Build history of the part. All positions in model axes, mm. Give positions to 0.01 mm unless a question says otherwise; leave off trailing zeros. Order: outer loops, then holes, each group sorted by start corner. A loop starts at its lowest first (then second) coordinate and runs counter-clockwise, first axis right, second up. Notation, with made-up numbers: (48.5, 20) - (63.5, 20) arc R14 cw to (63.5, 28) - close; hole circle Ø9 at (55, 76.25). An arc over 180 degrees is marked (long way). Answer in a Markdown table with one row per item.
```python
from build123d import *

# Parameters (mm, degrees)
SKETCH_1_W             = 5
SKETCH_1_H             = 3.6
EXTRUDE_1_DEPTH        = 50
CUT_EXTRUDE_1_DEPTH    = 101.047438748
SKETCH_3_R             = 1.79995
CUT_EXTRUDE_2_DEPTH    = 0.8
SKETCH_4_R             = 1.2
CUT_EXTRUDE_3_DEPTH    = 51.140702029
FILLET_1_R             = 0.3
FILLET_2_R             = 0.2
CHAMFER_1_SIZE         = 0.25
PATTERN_LINEAR_1_COUNT = 7
PATTERN_LINEAR_1_PITCH = 15


with BuildPart() as part:
    # 草图1 → 凸台-拉伸1 (new, symmetric)
    with BuildSketch(Plane(origin=(0, 0, 0), x_dir=(0, 0, -1), z_dir=(1, 0, 0))):
        Rectangle(SKETCH_1_W, SKETCH_1_H)
    extrude(amount=EXTRUDE_1_DEPTH, both=True)

    # 草图2 → 切除-拉伸1 (cut, through all)
    with BuildSketch(Plane(origin=(50, 0, 0), x_dir=(0, 0, -1), z_dir=(1, 0, 0))):
        with BuildLine():
            Line((2.5, 1.4), (2.5, 0.184))
            ThreePointArc((2.5, 0.184), (2.260324923, 0.318670305), (2.1, 0.542))
            Line((2.1, 0.542), (2, 0.542))
            ThreePointArc((2, 0.542), (1.75, 0.792), (2, 1.042))
            Line((2, 1.042), (2.1, 1.042))
            ThreePointArc((2.1, 1.042), (2.260324923, 1.265329695), (2.5, 1.4))
        make_face()
        with BuildLine():
            Line((-2.1, 1.042), (-2, 1.042))
            ThreePointArc((-2, 1.042), (-1.75, 0.792), (-2, 0.542))
            Line((-2, 0.542), (-2.1, 0.542))
            ThreePointArc((-2.1, 0.542), (-2.260324923, 0.318670305), (-2.5, 0.184))
            Line((-2.5, 0.184), (-2.5, 1.4))
            ThreePointArc((-2.5, 1.4), (-2.260324923, 1.265329695), (-2.1, 1.042))
        make_face()
    extrude(amount=-CUT_EXTRUDE_1_DEPTH, mode=Mode.SUBTRACT)

    # 草图3 → 切除-拉伸2 (cut)
    with BuildSketch(Plane(origin=(0, 1.8, 0), x_dir=(1, 0, 0), z_dir=(0, 1, 0))):
        with Locations(Location((-45, 0, 0), (0, 0, 270))):
            Circle(SKETCH_3_R)
    cut_extrude_2 = extrude(amount=-CUT_EXTRUDE_2_DEPTH, mode=Mode.SUBTRACT)

    # 草图4 → 切除-拉伸3 (cut, through all)
    with BuildSketch(Plane(origin=(0, 1, 0), x_dir=(1, 0, 0), z_dir=(0, 1, 0))):
        with Locations(Location((-45, 0, 0), (0, 0, 270))):
            Circle(SKETCH_4_R)
    cut_extrude_3 = extrude(amount=-CUT_EXTRUDE_3_DEPTH, mode=Mode.SUBTRACT)

    # 圆角1
    fillet_1_edges = [part.edges().sort_by_distance(p)[0] for p in [
        (0, 1.8, 2.5),
        (0, 1.8, -2.5),
    ]]
    fillet(fillet_1_edges, radius=FILLET_1_R)

    # 圆角2
    fillet_2_edges = [part.edges().sort_by_distance(p)[0] for p in [
        (0, 1.4, -2.5),
        (0, 1.042, -2.1),
        (0, 0.542, -2.1),
        (0, 0.184, -2.5),
        (0, 0.184, 2.5),
        (0, 1.4, 2.5),
        (0, 1.042, 2.1),
        (0, 0.542, 2.1),
    ]]
    fillet(fillet_2_edges, radius=FILLET_2_R)

    # 倒角1
    chamfer_1_edges = [part.edges().sort_by_distance(p)[0] for p in [
        (0, -1.8, -2.5),
        (0, -1.8, 2.5),
    ]]
    chamfer(chamfer_1_edges, length=CHAMFER_1_SIZE)

    # 阵列(线性)1: 切除-拉伸2, 切除-拉伸3 ×7
    with Locations(*[(i * PATTERN_LINEAR_1_PITCH, 0, 0) for i in range(1, PATTERN_LINEAR_1_COUNT)]):
        add(cut_extrude_2, mode=Mode.SUBTRACT)
        add(cut_extrude_3, mode=Mode.SUBTRACT)


solid = part.part
```
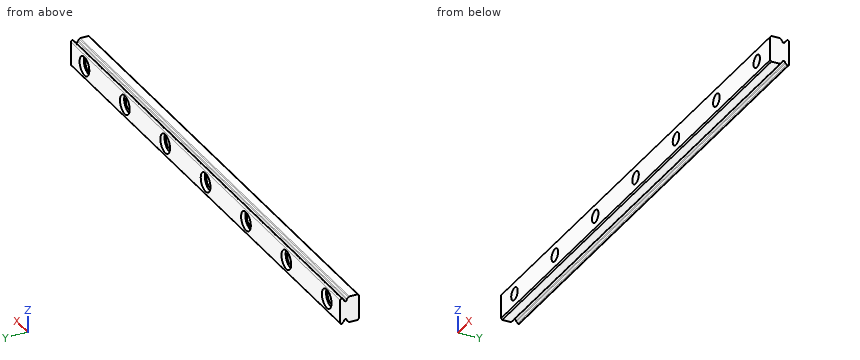
1. Drop flat-ended pins along their axis: P1, Ø1.4, axis at x = 0, z = 0, coming from the -Y side; P2, Ø3, axis at x = 0, z = 0, coming from the +Y side. Give the stop position or say it passes through.
Check result:
| item | result |
|---|---|
| P1 | passes through |
| P2 | stops at y = 1 |
2. Cut at B-B on z = 0.1. Count the separate pieces of the cut face and the enclosed holes in it, and give its area (3 significant figures).
Check result:
| item | result |
|---|---|
| separate pieces | 8 |
| enclosed holes | 0 |
| area | 293 mm² |
3. Cut at A-A on y = -0.55. Write the cut outline in (x, z), and give its area (3 significant figures).
Check result:
| item | result |
|---|---|
| outline | (-50, -2.5) - (50, -2.5) - (50, 2.5) - (-50, 2.5) - close; hole circle Ø2.4 at (-45, 0); hole circle Ø2.4 at (-30, 0); hole circle Ø2.4 at (-15, 0); hole circle Ø2.4 at (0, 0); hole circle Ø2.4 at (15, 0); hole circle Ø2.4 at (30, 0); hole circle Ø2.4 at (45, 0) |
| area | 468 mm² |
4. Probe line 1 (Y direction, x = -6.5, z = -2.05); line 2 (Z direction, x = 26.5, y = 0.8); line 3 (Z direction, x = 0.5, y = -1.55). List the from-to ranges inside material, lowest first.
Check result:
| item | result |
|---|---|
| line 1 | y = -1.8 to 0.53, 1.05 to 1.8 |
| line 2 | z = -1.75 to 1.75 |
| line 3 | z = -2.5 to -1.09, 1.09 to 2.5 |
